Design review of the part built by this model. Coordinates are the model's own, in mm. A direction names the side the tool comes from. Coordinates: 2 decimals unless noted, no trailing zeros. Write each loop counter-clockwise with the first axis right and the second up, starting at its lowest first coordinate (ties: lowest second). Pieces come first, ordered by that corner, then holes. Notation, with made-up numbers: (39.5, 31) - (56.5, 31) arc R26 ccw to (56.5, 50) - close; hole circle Ø5 at (7, 72.25). An arc over 180 degrees is marked (long way). Answer as CSV lines item,"result". Start each with the question number.
Q1. Machinability: for faces 1 (the face through (-23.11, -63.47, 20)), 2 (the face through (-4.336, -0.688, 19.524)), 3 (the face through (0.86, 63.47, 79.08)), which of the approach directions +Z, -Z, +X, -X, +Y, -Y give a long, thin tool a straight path to every point of the face, cutting with its end or side? Answer none if there is none.
Q2. We need section B-B (x = 30). Write out the cut boundary in (y, z), plus the area to 3 significant figures.
Q3. Mouldability with a two-part tool opening along X and no side actions: class faces 4 (the face through (75.285, 63.528, 31.215)), 5 (the face through (31.996, -63.472, -1.038)), 6 (the face through (-64.49, 63.47, 38.01)), 7 (the face through (-19, 61.5, -17)) as pulls with the +X half, pulls with the -X half, needs draft (parallel to the pull), parting line crosses it, or undercut.
Q4. For line 1 along Y through (x, z) = (-16, -21); line 2 along Y through (x, z) = (-36, -64); line 3 along X through (y, z) = (63.8, -38.5), list the stretches that pass through material, from the lowest coordinate up. Write a range as [from, to].
Q5. We need section A-A (z = 0). Write out the cut boundary in (x, y).
Q6. We need section D-D (z = -38.5). Write out the cut boundary in (x, y).
Q7. We need section C-C (z = 77). Write out the cut boundary in (x, y).
Q8. Clearance check with flat-ended pins moving along their axes: pin 1 (4 mm diameter, centred on x = 0, z = -77, fed in from -Y); pin 2 (1.5 mm diameter, centred on x = 42, z = -22, fed in from -Y). State where each tip first meets the part, or that it passes through.
Autodesk Inventor part; units mm, degrees
ref_plane "YZ Plane" through (0, 0, 0) normal (1, 0, 0) x (0, 1, 0)
ref_plane "XZ Plane" through (0, 0, 0) normal (0, 1, 0) x (-1, 0, 0)
ref_plane "XY Plane" through (0, 0, 0) normal (0, 0, 1) x (1, 0, 0)
sketch "Sketch1" plane through (0, 0, 0) normal (0, 0, 1) x (1, 0, 0)
  line L0 (0, 91.7) -> (0, -91.7) construction
  line L1 (-16.3, 0) -> (97.8, 0) construction
  line L2 (0, -65.5) -> (0, 65.5)
  line L3 (0, -65.5) -> (81.5, -65.5)
  line L4 (81.5, -65.5) -> (81.5, 65.5)
  line L5 (81.5, 65.5) -> (0, 65.5)
  point P0 (0, 0)
  dimension "d2" = 131
  dimension "d12" = 81.5
revolve "Revolution1" add sketch "Sketch1" angle 360 about axis through (0, 0, 0) along (0, -1, 0)
sketch "Sketch4" plane through (0, 0, 0) normal (0, 0, 1) x (1, 0, 0)
  line L0 (-81.5, 65.5) -> (81.5, 65.5) construction
  line L1 (-81.5, -65.5) -> (81.5, -65.5) construction
  line L2 (0, 91) -> (0, -91) construction
  line L3 (-114.1, 0) -> (114.1, 0) construction
  line L4 (35, -61.5) -> (22, -61.5)
  line L5 (20, -59.5) -> (20, 56.5)
  line L6 (25, 61.5) -> (81.5, 61.5)
  line L7 (81.5, 65.5) -> (81.5, -65.5) construction
  line L8 (81.5, -65.5) -> (81.5, 61.5)
  arc A0 (20, -59.5) -> (22, -61.5) centre (22, -59.5) ccw
  arc A1 (25, 61.5) -> (20, 56.5) centre (25, 56.5) ccw
  line L9 (35, -65.5) -> (35, -61.5)
  line L10 (-81.5, -65.5) -> (81.5, -65.5) construction
  line L11 (35, -65.5) -> (81.5, -65.5)
  point P0 (0, 0)
  dimension "d35" = 20
  dimension "d36" = 4
  dimension "d37" = 2
  dimension "d39" = 35
  dimension "d40" = 5
revolve "Revolution2" cut sketch "Sketch4" angle 360 about axis through (0, 0, 0) along (0, -1, 0)
sketch "Sketch2" plane through (0, -65.5, 0) normal (0, -1, 0) x (1, 0, 0)
  circle A0 centre (0, 0) radius 81.5 construction
  line L0 (-114.1, 0) -> (114.1, 0) construction
  line L1 (0, 114.1) -> (0, -114.1) construction
  circle A1 centre (0, 0) radius 21.25 construction
  circle A2 centre (0, 0) radius 30 construction
  point P0 (0, 30)
  point P1 (0, 21.25)
  point P2 (-21.2132, 21.2132)
  point P3 (-15.026, 15.026)
  point P4 (-30, 0)
  point P5 (-21.25, 0)
  point P6 (-21.2132, -21.2132)
  point P7 (-15.026, -15.026)
  point P8 (0, -30)
  point P9 (0, -21.25)
  point P10 (21.2132, -21.2132)
  point P11 (15.026, -15.026)
  point P12 (30, 0)
  point P13 (21.25, 0)
  point P14 (21.2132, 21.2132)
  point P15 (15.026, 15.026)
  point P16 (-4.5183, 21.1087)
  dimension "d6" = 42.5
  dimension "d7" = 60
  dimension "d10" = 360
hole "Hole2" at (0, -65.5, 30) at (-21.2132, -65.5, 21.2132) at (-30, -65.5, 0) at (-21.2132, -65.5, -21.2132) at (0, -65.5, -30) at (21.2132, -65.5, -21.2132) at (30, -65.5, 0) at (21.2132, -65.5, 21.2132) direction (0, 1, 0) diameter 4.5 depth 4
sketch "Sketch5" plane through (0, 65.5, 0) normal (0, 1, 0) x (1, 0, 0)
  line L0 (0, 114.1) -> (0, -114.1) construction
  line L1 (114.1, 0) -> (-114.1, 0) construction
  circle A0 centre (0, 0) radius 77 construction
  point P0 (0, 77)
  point P1 (-66.684, 38.5)
  point P2 (-66.684, -38.5)
  point P3 (0, -77)
  point P4 (66.684, -38.5)
  point P5 (66.684, 38.5)
  dimension "d45" = 154
  dimension "d43" = 360
hole "Hole3" at (0, 65.5, -77) at (-66.684, 65.5, -38.5) at (-66.684, 65.5, 38.5) at (0, 65.5, 77) at (66.684, 65.5, 38.5) at (66.684, 65.5, -38.5) direction (0, -1, 0) diameter 4.5 depth 4
properties part number "Connection_link_1"
Results list:
1,face 1,"-Y"
1,face 2,"none"
1,face 3,"+Y, -Y"
2,outline,"(-65.5, -18.03) - (-61.5, -18.03) - (-61.5, -2.25) - (-65.5, -2.25) - close; (-65.5, 2.25) - (-61.5, 2.25) - (-61.5, 18.03) - (-65.5, 18.03) - close; (61.5, -75.78) - (65.5, -75.78) - (65.5, 75.78) - (61.5, 75.78) - close"
2,area,"732 mm2"
3,face 4,"parting line crosses it"
3,face 5,"undercut"
3,face 6,"undercut"
3,face 7,"needs draft"
4,line 1,"y = [-65.5, -61.5], [61.5, 65.5]"
4,line 2,"y = [61.5, 65.5]"
4,line 3,"x = [-71.83, -68.93], [-64.43, 64.43], [68.93, 71.83]"
5,outline,"(-81.5, 61.5) - (-25, 61.5) arc R5 cw to (-20, 56.5) - (-20, -59.5) arc R2 cw to (-22, -61.5) - (-27.75, -61.5) - (-27.75, -65.5) - (27.75, -65.5) - (27.75, -61.5) - (22, -61.5) arc R2 cw to (20, -59.5) - (20, 56.5) arc R5 cw to (25, 61.5) - (81.5, 61.5) - (81.5, 65.5) - (-81.5, 65.5) - close; (-35, -65.5) - (-32.25, -65.5) - (-32.25, -61.5) - (-35, -61.5) - close; (32.25, -65.5) - (35, -65.5) - (35, -61.5) - (32.25, -61.5) - close"
6,outline,"(-71.83, 61.5) - (-68.93, 61.5) - (-68.93, 65.5) - (-71.83, 65.5) - close; (-64.43, 61.5) - (64.43, 61.5) - (64.43, 65.5) - (-64.43, 65.5) - close; (68.93, 61.5) - (71.83, 61.5) - (71.83, 65.5) - (68.93, 65.5) - close"
7,outline,"(-26.71, 61.5) - (-2.25, 61.5) - (-2.25, 65.5) - (-26.71, 65.5) - close; (2.25, 61.5) - (26.71, 61.5) - (26.71, 65.5) - (2.25, 65.5) - close"
8,pin 1,"passes through"
8,pin 2,"stops at y = 61.5"
